Input: dimensioned drawing with shaded views. Units: mm. Origin: part minimum x, y, z. A direction names the side the tool comes from. Give positions to 0.01 mm unless a question says otherwise; leave off trailing zeros. Write each loop counter-clockwise with the first axis right and the second up, starting at its lowest first coordinate (ties: lowest second). Pieces come first, ordered by that corner, then holes. Notation, with made-up numbers: M -0.5,-37 L 49.5,-37 A29 cw 49.5,-1 Z; hole C 8,-37.75 d6. An arc over 180 degrees is marked long. Answer as a JSON object with one key per item and string values.
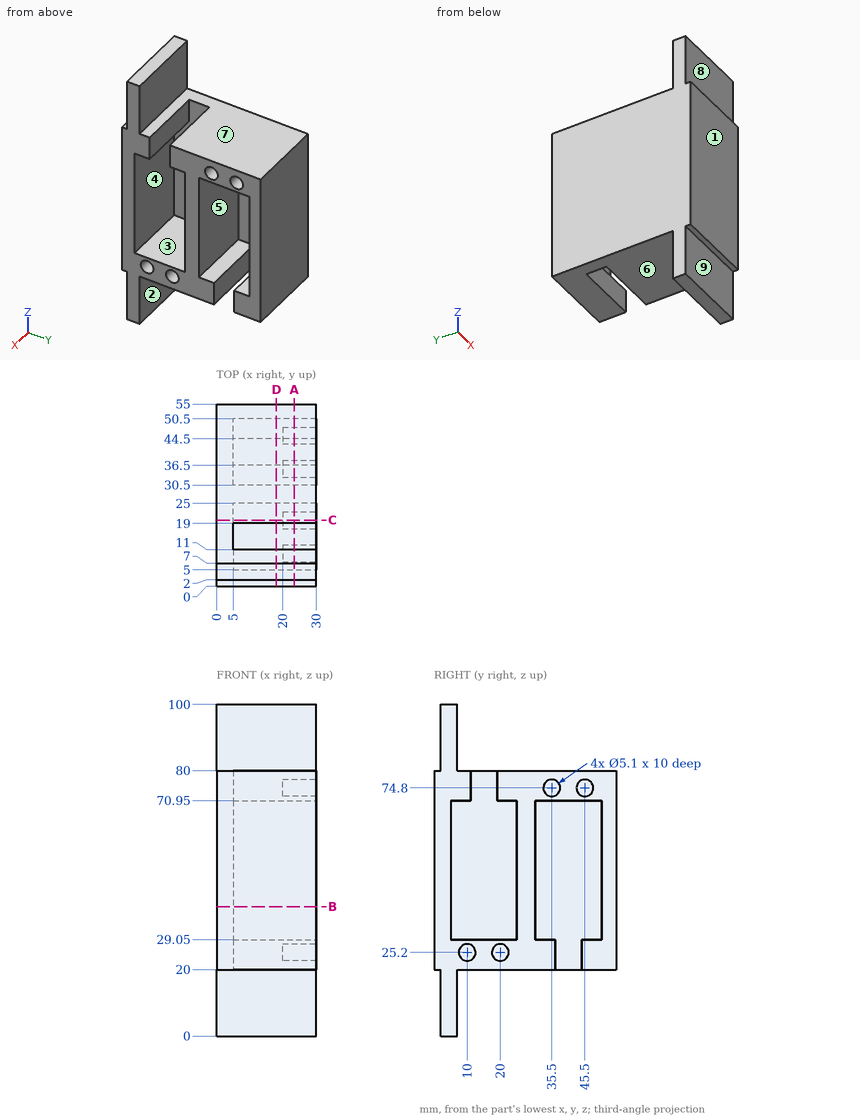
1) Contact query for flat-ended pins moving along their axis: P1, Ø6, axis at x = 20, y = 16.5, coming from the -Z side; P2, Ø1.5, axis at y = 41.5, z = 26, coming from the +X side; P3, Ø4, axis at y = 35.5, z = 74.8, coming from the +X side. Output: stop coordinate, or through.
Geometry check:
{"P1": "stops at z = 20", "P2": "stops at x = 5", "P3": "stops at x = 20"}
2) Line query: line 1 (Y direction, x = 24.5, z = 25.2); line 2 (Y direction, x = 21, z = 62.5); line 3 (Z direction, x = 13, y = 32). Output: solid intervals per line, ascending. Write a range as from..to.
Geometry check:
{"line 1": "y = 0..7.45, 12.55..17.45, 22.55..36.5, 44.5..55", "line 2": "y = 0..5, 25..30.5, 50.5..55", "line 3": "z = 20..29.05, 70.95..80"}
3) Pull-direction query (Y, two-part tool) for the marked faces 1, 2, 3 and 4; classes: pulls with the +Y half, pulls with the -Y half, needs draft (parallel to the pull), parting line crosses it, or undercut.
Geometry check:
{"face 1": "pulls with the -Y half", "face 2": "pulls with the +Y half", "face 3": "undercut", "face 4": "undercut"}
4) Cut plane A-A on x = 23.5. Give the number of separate pieces and of enclosed holes in the cut face, and give its area (3 significant figures).
Geometry check:
{"separate pieces": "1", "enclosed holes": "4", "area": "1,600 mm2"}
5) Set-up query: the marked faces 5, 6, 7, 8 and 9. Return all of +Z, -Z, +X, -X, +Y, -Y with unobstructed straight access to the full face (end or side cutting, diameter ignored); none if empty.
Geometry check:
{"face 5": "+X", "face 6": "-Z, +X, -X, +Y", "face 7": "+Z, +X, -X, +Y", "face 8": "+Z, +X, -X, -Y", "face 9": "-Z, +X, -X, -Y"}
6) Cut plane C-C on y = 20. Return loops of the section in (x, z), and give its area (4 significant figures).
Geometry check:
{"outline": "M 0,20 L 30,20 L 30,22.65 L 20,22.65 L 20,27.75 L 30,27.75 L 30,29.05 L 5,29.05 L 5,70.95 L 30,70.95 L 30,80 L 0,80 Z", "area": "701.5 mm2"}
7) Cut plane D-D on x = 18. Return loops of the section in (y, z), and give its area (3 significant figures).
Geometry check:
{"outline": "M 0,20 L 2,20 L 2,0 L 7,0 L 7,20 L 36.5,20 L 36.5,29.05 L 30.5,29.05 L 30.5,70.95 L 50.5,70.95 L 50.5,29.05 L 44.5,29.05 L 44.5,20 L 55,20 L 55,80 L 19,80 L 19,70.95 L 25,70.95 L 25,29.05 L 5,29.05 L 5,70.95 L 11,70.95 L 11,80 L 7,80 L 7,100 L 2,100 L 2,80 L 0,80 Z", "area": "1,680 mm2"}
8) Cut plane B-B on z = 39. Return loops of the section in (x, y), and give its area (3 significant figures).
Geometry check:
{"outline": "M 0,0 L 30,0 L 30,5 L 5,5 L 5,25 L 30,25 L 30,30.5 L 5,30.5 L 5,50.5 L 30,50.5 L 30,55 L 0,55 Z", "area": "650 mm2"}
